Build history of the part. All positions in model axes, mm. A direction names the side the tool comes from. Round coordinates to 2 decimals unless told otherwise and drop trailing zeros. Write each loop counter-clockwise with the first axis right and the second up, starting at its lowest first coordinate (ties: lowest second). Pieces come first, ordered by that corner, then holes. Notation, with made-up numbers: M 24,37.25 L 77,37.25 A11 ccw 77,58.25 Z; hole C -6,47 d4. An arc over 180 degrees is marked long. One line per item, written item: value. Start each with the question number.
```python
from build123d import *

# Parameters (mm, degrees)
BOSS_EXTRUDE1_DEPTH    = 1200
BOSS_EXTRUDE2_DEPTH    = 320
CUT_EXTRUDE2_START     = 0.5
SKETCH6_W              = 165
SKETCH6_H              = 60
CUT_EXTRUDE2_DEPTH     = 10
BOSS_EXTRUDE14_DEPTH   = 15
LPATTERN1_COUNT        = 2
LPATTERN1_PITCH        = 136
LPATTERN2_COUNT        = 2
LPATTERN2_PITCH        = 75
LPATTERN2_COPY_1_DEPTH = 15
CUT_EXTRUDE5_START     = 70
SKETCH14_R             = 2.5
CUT_EXTRUDE5_DEPTH     = 80
BOSS_EXTRUDE19_DEPTH   = 320
CUT_EXTRUDE10_DEPTH    = 320
BOSS_EXTRUDE20_DEPTH   = 320
CUT_EXTRUDE11_DEPTH    = 320
CUT_EXTRUDE12_DEPTH    = 320
SKETCH32_W             = 66.375164862
SKETCH32_H             = 1200
BOSS_EXTRUDE21_DEPTH   = 5
SKETCH33_W             = 219.088897638
SKETCH33_H             = 1200
BOSS_EXTRUDE23_DEPTH   = 5
SKETCH34_W             = 10
SKETCH34_H             = 70
BOSS_EXTRUDE24_DEPTH   = 30
CUT_EXTRUDE13_REACH    = 91.42
SKETCH35_W             = 18
SKETCH35_H             = 60


with BuildPart() as part:
    # Sketch1 → Boss-Extrude1 (new body)
    with BuildSketch(Plane(origin=(0, 0, 0), x_dir=(1, 0, 0), z_dir=(0, 1, 0))):
        Polygon((-138.29, -160), (-143.29, -160), (-143.29, 165), (144.1740625, 165), (144.1740625, -160), (138.29, -160), (138.29, 160), (-138.29, 160), align=None)
    extrude(amount=BOSS_EXTRUDE1_DEPTH)

    # Sketch3 → Boss-Extrude2 (add)
    with BuildSketch(Plane.XY.offset(-160)):
        Polygon((138.29, 50), (-138.29, 178.971372093), (-138.29, 188.971372093), (138.29, 60), align=None)
    extrude(amount=BOSS_EXTRUDE2_DEPTH)

    # Sketch6 → Cut-Extrude2 (cut)
    with BuildSketch(Plane(origin=(47.680784022, 102.25177131, 0), x_dir=(0.906307787, -0.422618262, 0), z_dir=(0.422618262, 0.906307787, 0)).offset(CUT_EXTRUDE2_START)):
        with Locations((-3.631700195, 0)):
            Rectangle(SKETCH6_W, SKETCH6_H)
    extrude(amount=-CUT_EXTRUDE2_DEPTH, mode=Mode.SUBTRACT)

    # Sketch15 → Boss-Extrude14 (add)
    with BuildSketch(Plane.XY.offset(-30)):
        Polygon((-30.960803737, 128.922945932), (-12.411066849, 120.273061564), (-12.411066849, 105.273061564), (-30.960803737, 113.922945932), align=None)
    boss_extrude14 = extrude(amount=-BOSS_EXTRUDE14_DEPTH)

    # LPattern1: Boss-Extrude14 ×2
    with Locations(*[Vector(0.906307787, -0.422618262, 0) * (i * LPATTERN1_PITCH) for i in range(1, LPATTERN1_COUNT)]):
        add(boss_extrude14)

    # LPattern2: Boss-Extrude14 ×2
    with Locations(*[(0, 0, i * LPATTERN2_PITCH) for i in range(1, LPATTERN2_COUNT)]):
        add(boss_extrude14)

    # LPattern2 copy 1 sketch → LPattern2 copy 1 (add)
    with BuildSketch(Plane(origin=(123.257859037, -57.476083597, 45), x_dir=(1, 0, 0), z_dir=(0, 0, 1))):
        Polygon((-30.960803737, 128.922945932), (-12.411066849, 120.273061564), (-12.411066849, 105.273061564), (-30.960803737, 113.922945932), align=None)
    extrude(amount=-LPATTERN2_COPY_1_DEPTH)

    # Sketch14 → Cut-Extrude5 (cut)
    with BuildSketch(Plane.XY.offset(-30).offset(CUT_EXTRUDE5_START)):
        with Locations((-22.522311936, 121.195788594)):
            Circle(SKETCH14_R)
        with Locations((100.735547101, 63.719704997)):
            Circle(SKETCH14_R)
    extrude(amount=-CUT_EXTRUDE5_DEPTH, mode=Mode.SUBTRACT)

    # Sketch19 → Boss-Extrude19 (add)
    with BuildSketch(Plane.XY.offset(-160)):
        Polygon((82.798897638, 85.875925991), (82.798897638, 1200), (77.798897638, 1200), (77.798897638, 88.207464282), align=None)
    extrude(amount=BOSS_EXTRUDE19_DEPTH)

    # Sketch27 → Cut-Extrude10 (cut)
    with BuildSketch(Plane.XY.offset(160)):
        Polygon((77.798897638, 97.590680412), (82.798897638, 95.259142121), (82.798897638, 85.875925991), (77.798897638, 88.715225589), align=None)
    extrude(amount=-CUT_EXTRUDE10_DEPTH, mode=Mode.SUBTRACT)

    # Sketch28 → Boss-Extrude20 (add)
    with BuildSketch(Plane.XY.offset(160)):
        Polygon((77.798897638, 97.590680412), (83.146994647, 87.403232752), (82.798897638, 95.259142121), align=None)
    extrude(amount=-BOSS_EXTRUDE20_DEPTH)

    # Sketch29 → Cut-Extrude11 (cut)
    with BuildSketch(Plane.XY.offset(160)):
        Polygon((138.29, 60), (138.29, 63), (144.1740625, 61.2), (144.1740625, 60), align=None)
    extrude(amount=-CUT_EXTRUDE11_DEPTH, mode=Mode.SUBTRACT)

    # Sketch31 → Cut-Extrude12 (cut)
    with BuildSketch(Plane.XY.offset(160)):
        Polygon((77.798897638, 88.207464282), (82.798897638, 85.875925991), (77.798897638, 88.715225589), align=None)
    extrude(amount=-CUT_EXTRUDE12_DEPTH, mode=Mode.SUBTRACT)

    # Sketch32 → Boss-Extrude21 (add)
    with BuildSketch(Plane.XY.offset(160)):
        with Locations((110.986480069, 600)):
            Rectangle(SKETCH32_W, SKETCH32_H)
    extrude(amount=BOSS_EXTRUDE21_DEPTH)

    # Sketch33 → Boss-Extrude23 (add)
    with BuildSketch(Plane.XY.offset(160)):
        with Locations((-33.745551181, 600)):
            Rectangle(SKETCH33_W, SKETCH33_H)
    extrude(amount=BOSS_EXTRUDE23_DEPTH)

    # Sketch34 → Boss-Extrude24 (add)
    with BuildSketch(Plane(origin=(0, 0, 160), x_dir=(-1, 0, 0), z_dir=(0, 0, -1))):
        with Locations((-59.754002279, 503.393533755)):
            Rectangle(SKETCH34_W, SKETCH34_H)
    extrude(amount=-BOSS_EXTRUDE24_DEPTH)

    # Sketch35 → Cut-Extrude13 (cut, up to next)
    with BuildSketch(Plane.ZY.offset(-54.754002279), mode=Mode.PRIVATE) as cut_extrude13_sk1:
        with Locations((174, 503.393533755)):
            Rectangle(SKETCH35_W, SKETCH35_H)
    cut_extrude13_tool1 = extrude(cut_extrude13_sk1.sketch, amount=-CUT_EXTRUDE13_REACH, mode=Mode.PRIVATE) & part.part
    add(cut_extrude13_tool1.solids().sort_by_distance((54.754002, 503.393534, 174))[0], mode=Mode.SUBTRACT)


solid = part.part
```
Item 1: Cut at C-C, the plane y = 653.5. Write the cut outline in (x, z), plus the area to 3 significant figures.
Item 2: Cut at B-B, the plane x = 23. Write the cut outline in (y, z), plus the area to 3 significant figures.
Item 3: Cut at A-A, the plane z = 126.5. Write the cut outline in (x, y).
Item 4: Drill centre lines: line 1 (X direction, y = 474.5, z = -48); line 2 (Z direction, x = 104.5, y = 734.5); line 3 (X direction, y = 165, z = -127). Where is each one in solid material? Low to high.
Item 5: Two-plate mould, pull along Z, no slides. Class faces 1 (the flat face through (-2, 592, -165)), 2 (the flat face through (77.799, 725, 0)), 3 (the flat face through (111, 608, 165)), 4 (the flat face through (138.29, 25, 2)): pulls with the +Z half, pulls with the -Z half, needs draft (parallel to the pull), parting line crosses it, or undercut.
Item 6: Which spindle directions (+Z, -Z, +X, -X, +Y, -Y) get a long thin tool onto all of the face, cutting with end or side? Do faces 5 (the flat face through (-143.29, 592, -2)), 6 (the flat face through (-57, 71, 160)), 7 (the flat face through (-30, 652, 160)). Say none if no direction does.
Item 7: Cut at D-D, the plane x = -116. Write the cut outline in (y, z), plus the area to 3 significant figures.
Item 8: Drop flat-ended pins along their axis: pin 1 (10 mm diameter, centred on x = -82, z = 73, fed in from +Y); pin 2 (1 mm diameter, centred on x = -23.5, y = 1027.5, fed in from +Z); pin 3 (4 mm diameter, centred on x = 43, z = -93, fed in from +Y). Give the stop position or say it passes through.
Computed values:
1. outline: M -143.29,-165 L 144.17,-165 L 144.17,165 L 77.8,165 L 77.8,-160 L -138.29,-160 L -138.29,160 L 75.8,160 L 75.8,165 L -143.29,165 Z; hole M 82.8,-160 L 138.29,-160 L 138.29,160 L 82.8,160 Z
1. area: 7,950 mm2
2. outline: M 0,-165 L 1200,-165 L 1200,-160 L 113.76,-160 L 113.76,-30 L 103.76,-30 L 103.76,-160 L 0,-160 Z; M 0,160 L 103.76,160 L 103.76,30 L 113.76,30 L 113.76,160 L 1200,160 L 1200,165 L 0,165 Z
2. area: 14,600 mm2
3. outline: M -143.29,0 L -138.29,0 L -138.29,178.97 L 138.29,50 L 138.29,0 L 144.17,0 L 144.17,60 L 138.29,60 L -138.29,188.97 L -138.29,1200 L -143.29,1200 Z; M 77.8,97.59 L 83.15,87.4 L 82.8,95.26 L 82.8,1200 L 77.8,1200 Z; M 138.29,63 L 144.17,61.2 L 144.17,1200 L 138.29,1200 Z
4. line 1: x = -143.29 to -138.29, 77.8 to 82.8, 138.29 to 144.17
4. line 2: z = -165 to -160, 160 to 165
4. line 3: x = -143.29 to -138.29, -108.33 to -86.88, 77.8 to 82.8, 138.29 to 144.17
5. face 1: pulls with the -Z half
5. face 2: needs draft
5. face 3: pulls with the +Z half
5. face 4: undercut
6. face 5: +Z, -Z, -X, +Y, -Y
6. face 6: -Y
6. face 7: +Y
7. outline: M 0,-165 L 1200,-165 L 1200,-160 L 178.58,-160 L 178.58,160 L 1200,160 L 1200,165 L 0,165 L 0,160 L 168.58,160 L 168.58,-160 L 0,-160 Z
7. area: 15,200 mm2
8. pin 1: stops at y = 165.05
8. pin 2: stops at z = 165
8. pin 3: stops at y = 105.37
